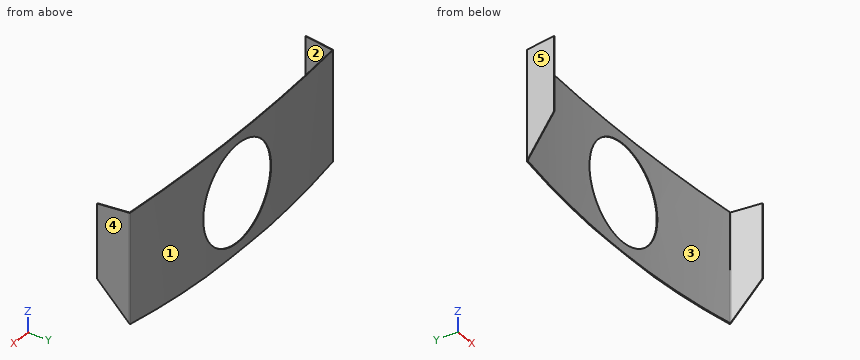
Autodesk Inventor part; units mm, degrees
ref_plane "YZ Plane" through (0, 0, 0) normal (1, 0, 0) x (0, 1, 0)
ref_plane "XZ Plane" through (0, 0, 0) normal (0, 1, 0) x (-1, 0, 0)
ref_plane "XY Plane" through (0, 0, 0) normal (0, 0, 1) x (1, 0, 0)
sketch "Sketch1" plane through (0, 0, 0) normal (0, 0, 1) x (1, 0, 0)
  line L0 (-785, -32) -> (785, -32) construction
  line L1 (785, -32) -> (785, 0) construction
  line L2 (785, 0) -> (-785, 0) construction
  line L3 (-785, 0) -> (-785, -32) construction
  arc A0 (745, -32) -> (-745, -32) centre (0, -8688.2656) ccw
  arc A1 (-745, -32) -> (-747.7174, -34.6) centre (-744.7428, -34.989) ccw
  line L4 (-747.7174, -34.6) -> (-767.2314, -183.8295)
  arc A2 (747.7174, -34.6) -> (745, -32) centre (744.7428, -34.989) ccw
  line L5 (747.7174, -34.6) -> (767.2314, -183.8295)
  line L6 (0, 0) -> (0, -32) construction
  dimension "d0" = 1570
  dimension "d1" = 32
  dimension "d2" = 40
  dimension "d14" = 3
  dimension "d15" = 150.5
  dimension "d16" = 97.45
  dimension "d21" = 8688.2656
contour flange "Contour Flange1" sketch "Sketch1" thickness 3 bend radius 3 width 600 along (0, 0, 1) mid plane no both sides no wall seen from (757.4744, -109.2147, 0) lies toward (0.9915584, 0.1296609, 0) curves L5 A2 A0 A1 L4
bend "Bend1"
corner "Corner1"
sketch "Sketch2" plane through (0, 0, 0) normal (1, 0, 0) x (0, 1, 0)
  line L0 (3, 0) -> (3, 600) construction
  line L1 (0, 600) -> (-183.8295, 380.9205)
  line L2 (3, 0) -> (-29.011, 0)
  line L3 (0, 0) -> (-183.8295, 219.0795)
  line L4 (-183.8295, 0) -> (-183.8295, 600)
  line L5 (3, 600) -> (-183.8295, 600)
  line L6 (-183.8295, 0) -> (3, 0)
  line L7 (0, 0) -> (-32, 0)
  line L8 (-32, 600) -> (0, 600)
  line L9 (0, 0) -> (0, 600) construction
  point P0 (-29.011, 0)
  point P1 (0, 0)
  dimension "d20" = 40
extrude "Extrusion1" cut sketch "Sketch2" along normal through all both and the other way through all contours L2 L6 L4 L3
sketch "Sketch3" plane through (0, 0, 0) normal (0, 1, 0) x (-1, 0, 0)
  circle A0 centre (0, 300) radius 250
  point P0 (0, 0)
  dimension "d22" = 500
  dimension "d25" = 300
extrude "Extrusion2" cut sketch "Sketch3" along normal through all both and the other way through all
equation "\"d14\" = BendRadius"
equation "\"d3\" = Thickness"
equation "\"d4\" = BendReliefWidth"
equation "\"d5\" = BendReliefDepth"
equation "\"d6\" = MinimumRemnant"
equation "\"d7\" = TransitionRadius"
equation "\"d9\" = BendRadius"
equation "\"d11\" = CornerReliefSize"
equation "\"d12\" = GapSize"
equation "\"d13\" = JacobiRadiusSize"
equation "\"BendRadius\" = Thickness"
equation "\"BendReliefWidth\" = Thickness"
equation "\"BendReliefDepth\" = 0.5 * Thickness"
equation "\"CornerReliefSize\" = 4 * Thickness"
equation "\"MinimumRemnant\" = 2 * Thickness"
equation "\"TransitionRadius\" = BendRadius"
equation "\"JacobiRadiusSize\" = BendRadius"
equation "\"GapSize\" = Thickness"
equation "\"Поясница_радиус\" = d21"
properties part number "МОО 031 лист  lowerback" material "Stainless Steel AISI 304"
Build history of the part. All positions in model axes, mm. Face numbers are marked on the shaded views. A direction names the side the tool comes from. Give positions to 0.01 mm unless a question says otherwise; leave off trailing zeros. Order: outer loops, then holes, each group sorted by start corner. A loop starts at its lowest first (then second) coordinate and runs counter-clockwise, first axis right, second up. Notation, with made-up numbers: M -14,31.25 L 11,31.25 A28 cw 11,70.25 Z; hole C 44.5,-20 d5. An arc over 180 degrees is marked long. Return JSON: item names as keys, results as strings.
Q1. Band-saw the part on B-B (z = 175.5). Give the cut face in (x, y).
Answer list:
{"outline": "M -765.48,-147.26 L -762.45,-147.26 L -747.72,-34.6 A3 cw -745,-32 A8688.27 cw -216.79,-2.71 L -216.79,0.3 A8691.27 ccw -745.26,-29.01 A6 ccw -750.69,-34.21 Z; M 216.79,-2.71 A8688.27 cw 745,-32 A3 cw 747.72,-34.6 L 762.45,-147.26 L 765.48,-147.26 L 750.69,-34.21 A6 ccw 745.26,-29.01 A8691.27 ccw 216.79,0.3 Z"}
Q2. 3-axis set-ups, long thin cutter, end or side, ignore diameter. For the marked faces 1 and 2: which of +Z, -Z, +X, -X, +Y, -Y reach the whole face in a straight line?
Answer list:
{"face 1": "+Z, -Z, +Y", "face 2": "+Z, -Z, -Y"}
Q3. Flat gauge pins, fed straight in: pin 1 (6 mm diameter, centred on y = -91.5, z = 166, fed in from +X); pin 2 (10 mm diameter, centred on x = -479.5, z = 133, fed in from -Y); pin 3 (4 mm diameter, centred on x = -254.5, z = 327, fed in from +Y). Where does each tip first touch, or does it go through?
Answer list:
{"pin 1": "stops at x = 758.58", "pin 2": "stops at y = -13.52", "pin 3": "stops at y = -0.67"}
Q4. Band-saw the part on A-A (y = -104). Give the cut face in (x, z), then the cut area to 3 significant figures.
Answer list:
{"outline": "M -759.82,123.94 L -756.79,123.94 L -756.79,600 L -759.82,600 Z; M 756.79,123.94 L 759.82,123.94 L 759.82,600 L 756.79,600 Z", "area": "2,880 mm^2"}
Q5. Band-saw the part on C-C (x = 107). Give the cut face in (y, z), then the cut area to 3 significant figures.
Answer list:
{"outline": "M -0.66,0.79 L 0,0 L 2.34,0 L 2.34,74.06 L -0.66,74.06 Z; M -0.66,525.94 L 2.34,525.94 L 2.34,600 L -0.66,600 Z", "area": "444 mm^2"}
Q6. Wall check: probe 1 along Z at (x, y) = (0, 1); probe 2 along X at (y, z) = (-152.5, 280.5); probe 3 along X at (y, z) = (-39, 487). Give the ranges that are in metal, low to high. Write a range as from..to.
Answer list:
{"probe 1": "z = 0..50, 550..600", "probe 2": "x = -766.16..-763.13, 763.13..766.16", "probe 3": "x = -751.32..-748.29, 748.29..751.32"}
Q7. Two-plate mould, pull along X, no slides. Class the marked faces 3, 4 and 5: pulls with the +X half, pulls with the -X half, needs draft (parallel to the pull), parting line crosses it, or undercut.
Answer list:
{"face 3": "undercut", "face 4": "pulls with the +X half", "face 5": "pulls with the -X half"}
Q8. Band-saw the part on D-D (z = 300). Give the cut face in (x, y).
Answer list:
{"outline": "M -770.21,-183.44 L -767.23,-183.83 L -747.72,-34.6 A3 cw -745,-32 A8688.27 cw -250,-3.6 L -250,-0.6 A8691.27 ccw -745.26,-29.01 A6 ccw -750.69,-34.21 Z; M 250,-3.6 A8688.27 cw 745,-32 A3 cw 747.72,-34.6 L 767.23,-183.83 L 770.21,-183.44 L 750.69,-34.21 A6 ccw 745.26,-29.01 A8691.27 ccw 250,-0.6 Z"}
